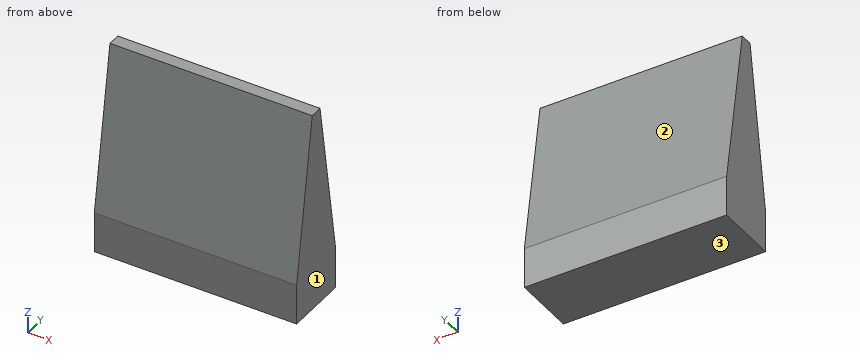
```python
from build123d import *

# Parameters (mm, degrees)
F0_W     = 160
F0_H     = 50
F1_DEPTH = 32
F3_DEPTH = 160


with BuildPart() as f1:
    # F0 (on Top) → F1 (new body)
    with BuildSketch(Plane.XY):
        Rectangle(F0_W, F0_H)
    extrude(amount=F1_DEPTH)

    # F2 (on face) → F3 (join)
    with BuildSketch(Plane(origin=(-80, 0, 0), x_dir=(0, -1, 0), z_dir=(-1, 0, 0))):
        Polygon((5, 160), (-5, 160), (-25, 32), (25, 32), align=None)
    extrude(amount=-F3_DEPTH)


solid = f1.part
```
Verification items for the finished model (mm, model axes). Face numbers are marked on the shaded views. Round coordinates to 2 decimals unless told otherwise and drop trailing zeros. Order: outer loops, then holes, each group sorted by start corner. A loop starts at its lowest first (then second) coordinate and runs counter-clockwise, first axis right, second up. Notation, with made-up numbers: (27, 17.5) - (36, 17.5) arc R19 ccw to (36, 28.5) - close; hole circle Ø10 at (31.5, 42.25). An arc over 180 degrees is marked (long way). Use CSV: the item, a comma, the result in double quotes. Start each with the question number.
1) Section check B-B, the plane y = -11. Record the cut outline in (x, z).
2) Go/stop test with a flat-tipped pin: P1, Ø2, axis at x = -57.5, z = 65.5, coming from the +Y side. Record where the tip stops, or that it passes through.
3) Mould release check, pull along Z, two halves, no side actions. Record for the marked faces 1, 2 and 3: +Z half, -Z half, draft (parallel to the pull), parting line (faces both ways), or undercut.
4) Section check C-C, the plane z = 110. Record the cut outline in (x, y), plus the area to 3 significant figures.
5) Section check A-A, the plane x = -45.5. Record the cut outline in (y, z).
6) Thickness scan on L1, parallel to Y at x = 57, z = 79.5; L2, parallel to Y at x = 15, z = 54.5. Record the ranges inside material, lowest first.
Answers:
1,outline,"(-80, 0) - (80, 0) - (80, 121.6) - (-80, 121.6) - close"
2,P1,"stops at y = 19.92"
3,face 1,"draft"
3,face 2,"+Z half"
3,face 3,"-Z half"
4,outline,"(-80, -12.81) - (80, -12.81) - (80, 12.81) - (-80, 12.81) - close"
4,area,"4,100 mm²"
5,outline,"(-25, 0) - (25, 0) - (25, 32) - (5, 160) - (-5, 160) - (-25, 32) - close"
6,L1,"y = -17.58 to 17.58"
6,L2,"y = -21.48 to 21.48"
